Could you check a few things on this model? Use its own coordinates, in mm. Round coordinates to 2 decimals unless told otherwise and drop trailing zeros. Write each loop counter-clockwise with the first axis right and the second up, starting at its lowest first coordinate (ties: lowest second). Pieces come first, ordered by that corner, then holes. Notation, with made-up numbers: M -15.5,-12 L 3.5,-12 A32 ccw 3.5,14 Z; hole C -2,26.5 d11. An arc over 180 degrees is marked long. One line per item, written item: value. Start each with the question number.
(1) I want a section at C-C on y = -2. Please give me the cut outline in (x, z).
(2) I want a section at B-B on x = 8. Please give me the cut outline in (y, z), and give its area (3 significant figures).
(3) I want a section at A-A on z = 2.75. Please give me the cut outline in (x, y), and give its area (3 significant figures).
(4) If I drill on L1, parallel to X at y = 2.75, z = 7.5; L2, parallel to Z at x = 5, y = -3.5; L3, parallel to Y at x = 6.5, z = 15.25, over which ranges is the centre line in solid material (lowest first)?
(5) I want a section at D-D on y = 10.5. Please give me the cut outline in (x, z), and give its area (3 significant figures).
(6) I'm going to push a flat-ended pin straight in: pin 1 Ø4 at (x, y) = (6.5, 8) entering from -Z. Where does the tip first touch, or does it pass through?
```python
from build123d import *

# Parameters (mm, degrees)
F0_W     = 25
F0_H     = 25
F1_DEPTH = 20
F2_R     = 5
F3_SIZE  = 10


with BuildPart() as f1:
    # F0 (on Top) → F1 (new body)
    with BuildSketch(Plane.XY):
        Rectangle(F0_W, F0_H)
    extrude(amount=F1_DEPTH)

    # F2
    f2_edges = [f1.edges().sort_by_distance(p)[0] for p in [
        (-12.5, 12.5, 10),
        (-12.5, 0, 20),
        (0, 12.5, 20),
    ]]
    fillet(f2_edges, radius=F2_R)

    # F3
    f3_edges = [f1.edges().sort_by_distance(p)[0] for p in [
        (12.5, 0, 0),
    ]]
    chamfer(f3_edges, length=F3_SIZE)


solid = f1.part
```
Found:
1. outline: M -12.5,0 L 2.5,0 L 12.5,10 L 12.5,20 L -7.5,20 A5 ccw -12.5,15 Z
2. outline: M -12.5,5.5 L 12.5,5.5 L 12.5,15 A5 ccw 7.5,20 L -12.5,20 Z
2. area: 357 mm²
3. outline: M -12.5,-12.5 L 5.25,-12.5 L 5.25,12.5 L -7.5,12.5 A5 ccw -12.5,7.5 Z
3. area: 438 mm²
4. L1: x = -12.5 to 10
4. L2: z = 2.5 to 20
4. L3: y = -12.5 to 12.49
5. outline: M -11.5,0 L 2.5,0 L 12.5,10 L 12.5,19 L -7.5,19 A4 ccw -11.5,15 Z
5. area: 403 mm²
6. pin 1: stops at z = 2
